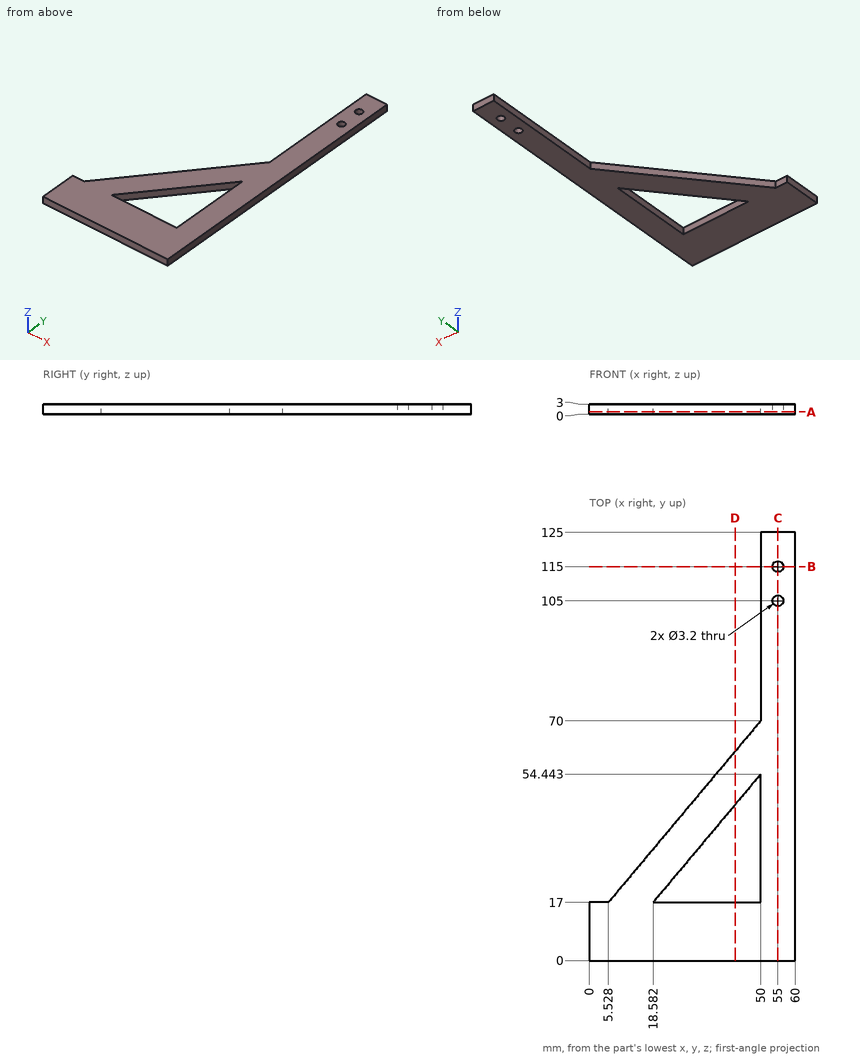
Geometry check sheet. Reference: drawing and pictorial views, mm from the part's lowest x, y, z. Give positions to 0.01 mm unless a question says otherwise; leave off trailing zeros. Write each loop counter-clockwise with the first axis right and the second up, starting at its lowest first coordinate (ties: lowest second). Pieces come first, ordered by that corner, then holes.
Item 1: Gauge pin test, flat ends, axial feed: pin 1 (0.9 mm diameter, centred on x = 39, z = 2, fed in from +Y); pin 2 (0.9 mm diameter, centred on y = 27, z = 1, fed in from -X); pin 3 (5 mm diameter, centred on x = 55, y = 115, fed in from +Z); pin 4 (0.9 mm diameter, centred on y = 84.5, z = 1, fed in from -X). Record the tip position at first contact, or that the pin passes through.
Item 2: Cross-section at B-B (y = 115). Enter the section's corners in (x, z).
Item 3: Cross-section at A-A (z = 0.7). Enter the section's corners in (x, y).
Item 4: Cross-section at D-D (x = 42.5). Enter the section's corners in (y, z) (1 decimal).
Item 5: Cross-section at C-C (x = 55). Enter the section's corners in (y, z), and give its area (3 significant figures).
Item 6: Scan lines: L1, parallel to Y at x = 55, z = 1.7; L2, parallel to X at y = 105, z = 0.85; L3, parallel to X at y = 71.5, z = 2.75. Record each from-to range of solid material in increasing order.
Report:
1. pin 1: stops at y = 57.43
1. pin 2: stops at x = 13.54
1. pin 3: stops at z = 3
1. pin 4: stops at x = 50
2. outline: (50, 0) - (53.4, 0) - (53.4, 3) - (50, 3) - close; (56.6, 0) - (60, 0) - (60, 3) - (56.6, 3) - close
3. outline: (0, 0) - (60, 0) - (60, 125) - (50, 125) - (50, 70) - (5.53, 17) - (0, 17) - close; hole (18.58, 17) - (50, 17) - (50, 54.44) - close; hole circle Ø3.2 at (55, 105); hole circle Ø3.2 at (55, 115)
4. outline: (0, 0) - (17, 0) - (17, 3) - (0, 3) - close; (45.5, 0) - (61.1, 0) - (61.1, 3) - (45.5, 3) - close
5. outline: (0, 0) - (103.4, 0) - (103.4, 3) - (0, 3) - close; (106.6, 0) - (113.4, 0) - (113.4, 3) - (106.6, 3) - close; (116.6, 0) - (125, 0) - (125, 3) - (116.6, 3) - close
5. area: 356 mm2
6. L1: y = 0 to 103.4, 106.6 to 113.4, 116.6 to 125
6. L2: x = 50 to 53.4, 56.6 to 60
6. L3: x = 50 to 60
